Could you check a few things on this model? Use its own coordinates, in mm. Give positions to 0.01 mm unless a question says otherwise; leave off trailing zeros. Loops run counter-clockwise (first coordinate to the right, second up) from the corner with the lowest first, then second, coordinate; pieces in that order, holes last. Notation, with made-up numbers: (0, -24) - (26, -24) arc R36 cw to (26, 14) - close; hole circle Ø7 at (81.5, 3.25). An arc over 180 degrees is marked (long way). Answer in a Markdown table with one row per item. Add a question column.
```python
from build123d import *

# Parameters (mm, degrees)
SKETCH_1_R               = 52.5
SKETCH_1_R_2             = 51
EXTRUDE_1_DEPTH          = 350
SKETCH_2_R               = 2
CUT_EXTRUDE_1_DEPTH      = 64
PATTERN_CIRCULAR_1_COUNT = 6


with BuildPart() as part:
    # Эскиз1 → Бобышка-Вытянуть1 (new body)
    with BuildSketch(Plane(origin=(0, 0, 0), x_dir=(1, 0, 0), z_dir=(0, 1, 0))):
        with Locations(Location((0, 0, 0), (0, 0, 270))):
            Circle(SKETCH_1_R)
        with Locations(Location((0, 0, 0), (0, 0, 270))):
            Circle(SKETCH_1_R_2, mode=Mode.SUBTRACT)
    extrude(amount=EXTRUDE_1_DEPTH)

    # Эскиз2 → Вырез-Вытянуть1 (cut)
    with BuildSketch(Plane.XY):
        with Locations(Location((0, 340, 0), (0, 0, 180))):
            Circle(SKETCH_2_R)
    cut_extrude_1 = extrude(amount=CUT_EXTRUDE_1_DEPTH, mode=Mode.SUBTRACT)

    # Круговой массив1: Вырез-Вытянуть1 ×6 about axis
    pattern_circular_1_axis = Axis((0, 350, 0), (0, -1, 0))
    for i in range(1, PATTERN_CIRCULAR_1_COUNT):
        add(cut_extrude_1.rotate(pattern_circular_1_axis, i * 360 / PATTERN_CIRCULAR_1_COUNT), mode=Mode.SUBTRACT)


solid = part.part
```
(1) I want a section at B-B on x = -23. Please give me the cut outline in (y, z), then the cut area to 3 significant figures.
(2) I want a section at C-C on y = 277.5. Please give me the cut outline in (x, z), then the cut area to 3 significant figures.
(3) For pin 1 Ø3 at (x, y) = (39, 91.5) entering from -Z; pin 2 Ø10 at (x, y) = (18, 235) entering from +Z (3 decimals); pin 3 Ø1.5 at (y, z) = (147.5, 2) entering from +X, each with a flat end and sliding along its axis, tell me the tip position at first contact or that it passes through.
(4) I want a section at A-A on z = 0. Please give me the cut outline in (x, y).
(5) Please list where these lines run through material, in increasing order: line 1 (Z direction, x = 0, y = 171); line 2 (Z direction, x = 7, y = 275.5); line 3 (X direction, y = 316, z = -30).
(6) We'd pull the mould along X, two halves only. Please class faces 1 (the cylindrical face through (-49.787, 172.55, -11.056)), 2 (the cylindrical face through (15.77, 172.55, 50.076)), 3 (the flat face through (8, 0, -51)): pulls with the +X half, pulls with the -X half, needs draft (parallel to the pull), parting line crosses it, or undercut.
Reported:
| question | item | result |
|---|---|---|
| 1 | outline | (0, -47.19) - (350, -47.19) - (350, -45.52) - (0, -45.52) - close; (0, 45.52) - (350, 45.52) - (350, 47.19) - (0, 47.19) - close |
| 1 | area | 1,170 mm² |
| 2 | outline | circle Ø105 at (0, 0); hole circle Ø102 at (0, 0) |
| 2 | area | 488 mm² |
| 3 | pin 1 | z = -36.74 |
| 3 | pin 2 | z = 50.865 |
| 3 | pin 3 | x = 52.49 |
| 4 | outline | (-52.5, 0) - (-51, 0) - (-51, 350) - (-52.5, 350) - close; (51, 0) - (52.5, 0) - (52.5, 350) - (51, 350) - close |
| 5 | line 1 | -52.5 to -51, 51 to 52.5 |
| 5 | line 2 | -52.03 to -50.52, 50.52 to 52.03 |
| 5 | line 3 | -43.08 to -41.24, 41.24 to 43.08 |
| 6 | face 1 | undercut |
| 6 | face 2 | parting line crosses it |
| 6 | face 3 | needs draft |
